The model under review builds one solid part; all positions refer to its coordinate system, in mm. Face numbers are marked on the shaded views. Coordinates: 2 decimals unless noted, no trailing zeros. Write each loop counter-clockwise with the first axis right and the second up, starting at its lowest first coordinate (ties: lowest second). Pieces come first, ordered by that corner, then holes. Notation, with made-up numbers: M 89,3.25 L 132,3.25 A19 ccw 132,31.25 Z; hole C 68.5,26.25 d11. An arc over 180 degrees is marked long. Answer as a JSON object with one key per item and string values.
Autodesk Inventor part; units mm, degrees
ref_plane "YZ Plane" through (0, 0, 0) normal (1, 0, 0) x (0, 1, 0)
ref_plane "XZ Plane" through (0, 0, 0) normal (0, 1, 0) x (-1, 0, 0)
ref_plane "XY Plane" through (0, 0, 0) normal (0, 0, 1) x (1, 0, 0)
sketch "Sketch1" plane through (0, 0, 0) normal (0, 1, 0) x (-1, 0, 0)
  line L0 (2.54, 0) -> (7.62, 0)
  line L1 (10.16, -2.54) -> (10.16, -17.78)
  line L2 (7.62, -20.32) -> (2.54, -20.32)
  line L3 (0, -17.78) -> (0, -2.54)
  arc A0 (10.16, -2.54) -> (7.62, 0) centre (7.62, -2.54) ccw
  arc A1 (7.62, -20.32) -> (10.16, -17.78) centre (7.62, -17.78) ccw
  arc A2 (0, -17.78) -> (2.54, -20.32) centre (2.54, -17.78) ccw
  arc A3 (2.54, 0) -> (0, -2.54) centre (2.54, -2.54) ccw
  circle A4 centre (7.62, -2.54) radius 1.27
  circle A5 centre (7.62, -17.78) radius 1.27
  point P0 (0, 0)
  point P1 (10.16, -20.32)
  point P2 (10.16, 0)
  point P3 (0, -20.32)
  dimension "d0" = 10.16
  dimension "d1" = 20.32
  dimension "d2" = 2.54
  dimension "d3" = 2.54
  dimension "d4" = 2.54
  dimension "d5" = 2.54
  dimension "d6" = 2.54
  dimension "d7" = 2.54
  dimension "d8" = 2.54
extrude "Extrusion1" add sketch "Sketch1" along normal blind 1.5748
properties part number "USB_Board"
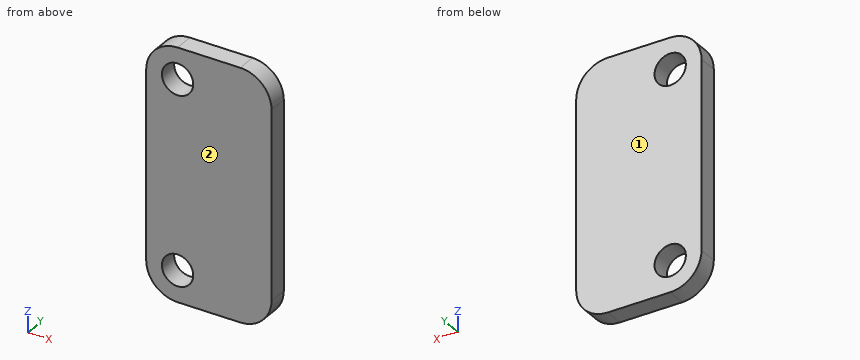
(1) For pin 1 Ø2 at (x, z) = (-7.62, -17.78) entering from -Y, flat-tipped, find the tip position at first contact; note if it passes through.
Results list:
{"pin 1": "through"}
(2) Add section A-A on y = 1.3. Give the boundary of the cut face in (x, z), and give its area (3 significant figures).
Results list:
{"outline": "M -10.16,-17.78 A2.54 ccw -7.62,-20.32 L -2.54,-20.32 A2.54 ccw 0,-17.78 L 0,-2.54 A2.54 ccw -2.54,0 L -7.62,0 A2.54 ccw -10.16,-2.54 Z; hole C -7.62,-17.78 d2.54; hole C -7.62,-2.54 d2.54", "area": "191 mm²"}
(3) Draft analysis for pull direction Y (two halves, no side actions). For the marked faces 1 and 2, state which applies: released by +Y, released by -Y, zero draft, split by the parting line, or undercut.
Results list:
{"face 1": "released by +Y", "face 2": "released by -Y"}
(4) Add section B-B on x = -7.25. Give the boundary of the cut face in (y, z).
Results list:
{"outline": "M 0,-20.32 L 1.57,-20.32 L 1.57,-18.99 L 0,-18.99 Z; M 0,-16.57 L 1.57,-16.57 L 1.57,-3.75 L 0,-3.75 Z; M 0,-1.33 L 1.57,-1.33 L 1.57,0 L 0,0 Z"}
(5) Add section C-C on z = -1.5. Give the boundary of the cut face in (x, y), and give its area (3 significant figures).
Results list:
{"outline": "M -9.94,0 L -8.35,0 L -8.35,1.57 L -9.94,1.57 Z; M -6.89,0 L -0.22,0 L -0.22,1.57 L -6.89,1.57 Z", "area": "13.0 mm²"}
(6) Wall thickness on line 1 along Z through (x, y) = (-7.62, 0.95); line 2 along Z through (x, y) = (-8.25, 0.4); line 3 along X through (y, z) = (1.25, -2.25): over which ranges is each line inside the solid? List them lowest first. Write a range as from..to.
Results list:
{"line 1": "-20.32..-19.05, -16.51..-3.81, -1.27..0", "line 2": "-20.24..-18.88, -16.68..-3.64, -1.44..-0.08", "line 3": "-10.14..-8.86, -6.38..-0.02"}
